Work out the finished part from the listing and answer in its coordinate system (mm). Face numbers are marked on the shaded views. Round coordinates to 2 decimals unless told otherwise and drop trailing zeros. Loops run counter-clockwise (first coordinate to the right, second up) from the corner with the lowest first, then second, coordinate; pieces in that order, holes last. Notation, with made-up numbers: (85.25, 72.5) - (111.25, 72.5) arc R20 ccw to (111.25, 109.5) - close; hole circle Ø10 at (-9.75, 58.25). An arc over 180 degrees is marked (long way). Return JSON: item names as keys, results as strings.
from build123d import *

# Parameters (mm, degrees)
SKETCH_R         = 5.5
PAD_DEPTH        = 3.17
HOLE_D           = 4.5
HOLE_DEPTH       = 25
HOLE_CSINK_D     = 6.3
HOLE_CSINK_ANGLE = 90
FILLET_R         = 1


with BuildPart() as part:
    # Sketch → Pad (new body)
    with BuildSketch(Plane.XY):
        with BuildLine():
            Line((-12.7, 8.1026), (-5.758899, 18.836875))
            ThreePointArc((5.758899, 18.836875), (0, 21.971), (-5.758899, 18.836875))
            Line((5.758899, 18.836875), (12.7, 8.1026))
            Line((12.7, 8.1026), (12.7, -8.1026))
            Line((12.7, -8.1026), (5.758899, -18.836875))
            ThreePointArc((-5.758899, -18.836875), (0, -21.971), (5.758899, -18.836875))
            Line((-5.758899, -18.836875), (-12.7, -8.1026))
            Line((-12.7, -8.1026), (-12.7, 8.1026))
        make_face()
        with Locations((2.5146, -3.2766)):
            Circle(SKETCH_R, mode=Mode.SUBTRACT)
    extrude(amount=-PAD_DEPTH)

    # Hole
    with Locations(Plane.XY):
        with Locations((0, 15.113), (0, -15.113)):
            CounterSinkHole(HOLE_D / 2, HOLE_CSINK_D / 2, depth=HOLE_DEPTH, counter_sink_angle=HOLE_CSINK_ANGLE)

    # Fillet
    fillet_edges = [part.edges().sort_by_distance(p)[0] for p in [
        (0, -21.971, 0),
        (12.7, 0, 0),
        (-12.7, 0, 0),
        (-9.22945, 13.469738, 0),
    ]]
    fillet(fillet_edges, radius=FILLET_R)


solid = part.part
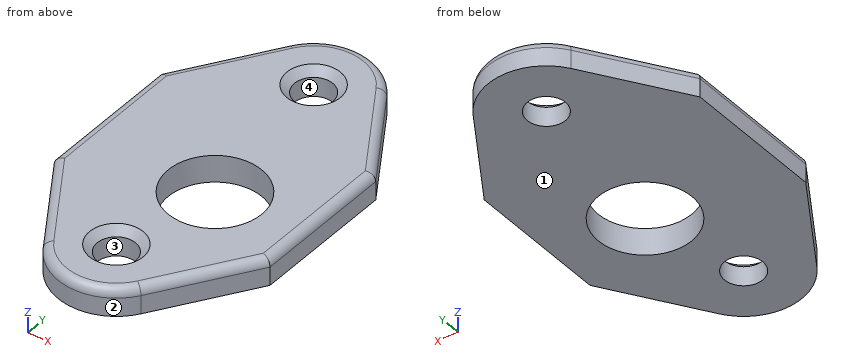
1) Section B-B (z = -2.2) is taken. Give the vertices of the cut face in (x, y), and give its area (3 significant figures).
Verdict:
{"outline": "(-12.7, -8.1) - (-5.76, -18.84) arc R6.86 ccw to (5.76, -18.84) - (12.7, -8.1) - (12.7, 8.1) - (5.76, 18.84) arc R6.86 ccw to (-5.76, 18.84) - (-12.7, 8.1) - close; hole circle Ø11 at (2.51, -3.28); hole circle Ø4.5 at (0, -15.11); hole circle Ø4.5 at (0, 15.11)", "area": "732 mm2"}
2) Flat-ended cylindrical pins translate along their axes: pin 1 (6 mm diameter, centred on x = 0, y = -15.113, fed in from +Z); pin 2 (10 mm diameter, centred on x = -0.5, y = -17, fed in from +Z). Find the tip coordinate at first contact, or state that the pin passes through.
Verdict:
{"pin 1": "stops at z = -0.15", "pin 2": "stops at z = 0"}
3) Find the intervals of material crossed by L1, parallel to Y at x = 1.5, z = -0.3; L2, parallel to Y at x = 0, z = -2.3; L3, parallel to X at y = 1, z = -2.7, in increasing order.
Verdict:
{"L1": "y = -21.51 to -17.54, -12.69 to -8.68, 2.13 to 12.69, 17.54 to 21.51", "L2": "y = -21.97 to -17.36, -12.86 to -8.17, 1.61 to 12.86, 17.36 to 21.97", "L3": "x = -12.7 to -0.94, 5.97 to 12.7"}
4) Determine the mould class of the marked faces 1, 2, 3 and 4 for opening direction X: pulls with the +X half, pulls with the -X half, needs draft (parallel to the pull), parting line crosses it, or undercut.
Verdict:
{"face 1": "needs draft", "face 2": "parting line crosses it", "face 3": "undercut", "face 4": "undercut"}
5) Section A-A (x = 0) is taken. Give the vertices of the cut face in (y, z), and give its area (3 significant figures).
Verdict:
{"outline": "(-21.97, -3.17) - (-17.36, -3.17) - (-17.36, -0.9) - (-18.26, 0) - (-20.97, 0) arc R1 ccw to (-21.97, -1) - close; (-12.86, -3.17) - (-8.17, -3.17) - (-8.17, 0) - (-11.96, 0) - (-12.86, -0.9) - close; (1.61, -3.17) - (12.86, -3.17) - (12.86, -0.9) - (11.96, 0) - (1.61, 0) - close; (17.36, -3.17) - (21.97, -3.17) - (21.97, -1) arc R1 ccw to (20.97, 0) - (18.26, 0) - (17.36, -0.9) - close", "area": "77.7 mm2"}
